```python
from build123d import *

# Parameters (mm, degrees)
F0_W         = 59
F0_H         = 140
F1_DEPTH     = 50
F2_R         = 5
F3_T1_DEPTH  = 130
F3_T3_DEPTH  = 49
F3_T5_DEPTH  = 59
F3_T7_DEPTH  = 140
F3_T10_ANGLE = 90
F3_T12_ANGLE = 90
F3_T14_ANGLE = 90
F3_T16_ANGLE = 90
F3_T18_ANGLE = 90
F3_T20_ANGLE = 90
F3_T22_ANGLE = 90
F3_T24_ANGLE = 90


# Not quite as in the source:
# - a fillet or chamfer that OpenCascade refuses, or shapes differently, is made with other operations: its cross-section is extruded or revolved along the edge and cut away or added


with BuildPart() as f1:
    # F0 (on Top) → F1 (new body)
    with BuildSketch(Plane.XY):
        with BuildLine():
            Line((-29.5, -72.5), (29.5, -72.5))
            ThreePointArc((29.5, -72.5), (31.267766953, -71.767766953), (32, -70))
            Line((32, -70), (32, 70))
            ThreePointArc((32, 70), (31.267766953, 71.767766953), (29.5, 72.5))
            Line((29.5, 72.5), (-29.5, 72.5))
            ThreePointArc((-29.5, 72.5), (-31.267766953, 71.767766953), (-32, 70))
            Line((-32, 70), (-32, -70))
            ThreePointArc((-32, -70), (-31.267766953, -71.767766953), (-29.5, -72.5))
        make_face()
        Rectangle(F0_W, F0_H, mode=Mode.SUBTRACT)
    extrude(amount=F1_DEPTH)

    # F2
    f2_edges = [f1.edges().sort_by_distance(p)[0] for p in [
        (-29.5, 70, 25),
        (29.5, 70, 25),
        (-29.5, -70, 25),
        (29.5, -70, 25),
    ]]
    fillet(f2_edges, radius=F2_R)

    # F3: fillet of radius 2 on 16 edges, made by hand

    # F3_s2 → F3_t1 (cut)
    with BuildSketch(Plane.XZ.offset(-65)):
        with BuildLine():
            ThreePointArc((29.5, 48), (30.0857864376, 49.4142135624), (31.5, 50))
            Line((31.5, 50), (29.5, 50))
            Line((29.5, 50), (29.5, 48))
        make_face()
        with BuildLine():
            ThreePointArc((-31.5, 50), (-30.0857864376, 49.4142135624), (-29.5, 48))
            Line((-29.5, 48), (-29.5, 50))
            Line((-29.5, 50), (-31.5, 50))
        make_face()
    extrude(amount=F3_T1_DEPTH, mode=Mode.SUBTRACT)

    # F3_s4 → F3_t3 (cut)
    with BuildSketch(Plane.YZ.offset(-24.5)):
        with BuildLine():
            ThreePointArc((72, 50), (70.5857864376, 49.4142135624), (70, 48))
            Line((70, 48), (70, 50))
            Line((70, 50), (72, 50))
        make_face()
        with BuildLine():
            ThreePointArc((-72, 50), (-70.5857864376, 49.4142135624), (-70, 48))
            Line((-70, 48), (-70, 50))
            Line((-70, 50), (-72, 50))
        make_face()
    extrude(amount=F3_T3_DEPTH, mode=Mode.SUBTRACT)

    # F3_s6 → F3_t5 (cut)
    with BuildSketch(Plane.YZ.offset(-29.5)):
        with BuildLine():
            ThreePointArc((-70.5, 50), (-71.9142135624, 49.4142135624), (-72.5, 48))
            Line((-72.5, 48), (-72.5, 50))
            Line((-72.5, 50), (-70.5, 50))
        make_face()
        with BuildLine():
            ThreePointArc((70.5, 50), (71.9142135624, 49.4142135624), (72.5, 48))
            Line((72.5, 48), (72.5, 50))
            Line((72.5, 50), (70.5, 50))
        make_face()
    extrude(amount=F3_T5_DEPTH, mode=Mode.SUBTRACT)

    # F3_s8 → F3_t7 (cut)
    with BuildSketch(Plane.XZ.offset(-70)):
        with BuildLine():
            ThreePointArc((30, 50), (31.4142135624, 49.4142135624), (32, 48))
            Line((32, 48), (32, 50))
            Line((32, 50), (30, 50))
        make_face()
        with BuildLine():
            ThreePointArc((-30, 50), (-31.4142135624, 49.4142135624), (-32, 48))
            Line((-32, 48), (-32, 50))
            Line((-32, 50), (-30, 50))
        make_face()
    extrude(amount=F3_T7_DEPTH, mode=Mode.SUBTRACT)

    # F3_s9 → F3_t10 (revolve, cut)
    with BuildSketch(Plane.XZ.offset(-65)):
        with BuildLine():
            ThreePointArc((29.5, 48), (30.0857864376, 49.4142135624), (31.5, 50))
            Line((31.5, 50), (29.5, 50))
            Line((29.5, 50), (29.5, 48))
        make_face()
    revolve(axis=Axis((24.5, 65, 50), (0, 0, 1)), revolution_arc=F3_T10_ANGLE, mode=Mode.SUBTRACT)

    # F3_s11 → F3_t12 (revolve, cut)
    with BuildSketch(Plane.XZ.offset(65)):
        with BuildLine():
            ThreePointArc((29.5, 48), (30.0857864376, 49.4142135624), (31.5, 50))
            Line((31.5, 50), (29.5, 50))
            Line((29.5, 50), (29.5, 48))
        make_face()
    revolve(axis=Axis((24.5, -65, 50), (0, 0, -1)), revolution_arc=F3_T12_ANGLE, mode=Mode.SUBTRACT)

    # F3_s13 → F3_t14 (revolve, cut)
    with BuildSketch(Plane.XZ.offset(-65)):
        with BuildLine():
            ThreePointArc((-31.5, 50), (-30.0857864376, 49.4142135624), (-29.5, 48))
            Line((-29.5, 48), (-29.5, 50))
            Line((-29.5, 50), (-31.5, 50))
        make_face()
    revolve(axis=Axis((-24.5, 65, 50), (0, 0, -1)), revolution_arc=F3_T14_ANGLE, mode=Mode.SUBTRACT)

    # F3_s15 → F3_t16 (revolve, cut)
    with BuildSketch(Plane.YZ.offset(-24.5)):
        with BuildLine():
            ThreePointArc((-72, 50), (-70.5857864376, 49.4142135624), (-70, 48))
            Line((-70, 48), (-70, 50))
            Line((-70, 50), (-72, 50))
        make_face()
    revolve(axis=Axis((-24.5, -65, 50), (0, 0, -1)), revolution_arc=F3_T16_ANGLE, mode=Mode.SUBTRACT)

    # F3_s17 → F3_t18 (revolve, cut)
    with BuildSketch(Plane.XZ.offset(70)):
        with BuildLine():
            ThreePointArc((-30, 50), (-31.4142135624, 49.4142135624), (-32, 48))
            Line((-32, 48), (-32, 50))
            Line((-32, 50), (-30, 50))
        make_face()
    revolve(axis=Axis((-29.5, -70, 50), (0, 0, 1)), revolution_arc=F3_T18_ANGLE, mode=Mode.SUBTRACT)

    # F3_s19 → F3_t20 (revolve, cut)
    with BuildSketch(Plane.YZ.offset(29.5)):
        with BuildLine():
            ThreePointArc((-70.5, 50), (-71.9142135624, 49.4142135624), (-72.5, 48))
            Line((-72.5, 48), (-72.5, 50))
            Line((-72.5, 50), (-70.5, 50))
        make_face()
    revolve(axis=Axis((29.5, -70, 50), (0, 0, 1)), revolution_arc=F3_T20_ANGLE, mode=Mode.SUBTRACT)

    # F3_s21 → F3_t22 (revolve, cut)
    with BuildSketch(Plane.XZ.offset(-70)):
        with BuildLine():
            ThreePointArc((30, 50), (31.4142135624, 49.4142135624), (32, 48))
            Line((32, 48), (32, 50))
            Line((32, 50), (30, 50))
        make_face()
    revolve(axis=Axis((29.5, 70, 50), (0, 0, 1)), revolution_arc=F3_T22_ANGLE, mode=Mode.SUBTRACT)

    # F3_s23 → F3_t24 (revolve, cut)
    with BuildSketch(Plane.YZ.offset(-29.5)):
        with BuildLine():
            ThreePointArc((70.5, 50), (71.9142135624, 49.4142135624), (72.5, 48))
            Line((72.5, 48), (72.5, 50))
            Line((72.5, 50), (70.5, 50))
        make_face()
    revolve(axis=Axis((-29.5, 70, 50), (0, 0, 1)), revolution_arc=F3_T24_ANGLE, mode=Mode.SUBTRACT)


solid = f1.part
```
Here's how the part is built. I have some questions about the finished solid (model axes, mm). A direction names the side the tool comes from. Round coordinates to 2 decimals unless told otherwise and drop trailing zeros. Loops run counter-clockwise (first coordinate to the right, second up) from the corner with the lowest first, then second, coordinate; pieces in that order, holes last.
1. Suppose I cut it at A-A, the plane x = -22.5. Please give me the cut outline in (y, z).
Answers:
outline: (-72.5, 0) - (-70, 0) - (-70, 48) arc R2 ccw to (-71.25, 49.85) arc R2 ccw to (-72.5, 48) - close; (70, 0) - (72.5, 0) - (72.5, 48) arc R2 ccw to (71.25, 49.85) arc R2 ccw to (70, 48) - close
2. If I drill on probe 1 along X at (y, z) = (21.5, 23.5); probe 2 along Y at (x, z) = (-14.5, 4); probe 3 along Y at (x, z) = (-28, 36), over which ranges is the centre line in solid material (lowest first)?
Answers:
probe 1: x = -32 to -29.5, 29.5 to 32
probe 2: y = -72.5 to -70, 70 to 72.5
probe 3: y = -72.5 to -68.57, 68.57 to 72.5
3. Suppose I cut it at C-C, the plane z = 11. Please give me the cut outline in (x, y).
Answers:
outline: (-32, -70) arc R2.5 ccw to (-29.5, -72.5) - (29.5, -72.5) arc R2.5 ccw to (32, -70) - (32, 70) arc R2.5 ccw to (29.5, 72.5) - (-29.5, 72.5) arc R2.5 ccw to (-32, 70) - close; hole (-29.5, -65) arc R5 ccw to (-24.5, -70) - (24.5, -70) arc R5 ccw to (29.5, -65) - (29.5, 65) arc R5 ccw to (24.5, 70) - (-24.5, 70) arc R5 ccw to (-29.5, 65) - close
4. Suppose I cut it at B-B, the plane y = 7. Please give me the cut outline in (x, z).
Answers:
outline: (-32, 0) - (-29.5, 0) - (-29.5, 48) arc R2 ccw to (-30.75, 49.85) arc R2 ccw to (-32, 48) - close; (29.5, 0) - (32, 0) - (32, 48) arc R2 ccw to (30.75, 49.85) arc R2 ccw to (29.5, 48) - close
5. Thinking about a two-plate mould opening in X: for faces 3 (the face through (32, -1, 24)), 4 (the face through (0, 72.5, 24)), 5 (the face through (0, -70, 24)), which applies, released by +X, released by -X, zero draft, split by the parting line, or undercut?
Answers:
face 3: released by +X
face 4: zero draft
face 5: undercut
6. For faces 1 (the face through (-31, 22, 0)), 2 (the face through (0, 70, 24)), which set-ups out of +Z, -Z, +X, -X, +Y, -Y let a thin tool reach every point of the face, with its end or its side?
Answers:
face 1: -Z, +X, -X, +Y, -Y
face 2: +Z, -Z
